Geometry: final body of the model. Coordinates: model frame, mm. Face numbers are marked on the shaded views. A direction names the side the tool comes from. Give positions to 0.01 mm unless a question says otherwise; leave off trailing zeros. Loops run counter-clockwise (first coordinate to the right, second up) from the corner with the lowest first, then second, coordinate; pieces in that order, holes last.
1. Section A-A, the plane y = 6. Output: boundary loops of the cut face in (x, z), then the cut area to 3 significant figures.
2. Section B-B, the plane y = -6.5. State how many separate pieces and enclosed holes the cut face has, then the cut area to 3 significant figures.
3. First-contact query: P1, Ø2, axis at y = -6, z = 19.5, coming from the +X side; P2, Ø15, axis at x = 0.5, z = -24.5, coming from the +Y side; P3, Ø1, axis at y = -6, z = -4, coming from the +X side. Flat tips, straight axial feed; report the tip coordinate or a pass-through.
4. Access query for the marked faces 1 and 2. Directions: +Z, -Z, +X, -X, +Y, -Y. A direction counts if a zero-diameter tool reaches every point of the face in a straight line with its end or side. Return the directions, or none.
5. Material intervals for line 1 along Z through (x, y) = (-6, 7); line 2 along X through (y, z) = (-7.5, 1.5); line 3 along X through (y, z) = (4.5, -15), sorted ascending.
6. Draft query along Y for the marked faces 3, 4, 5 and 6. Return one class per face: +Y half, -Y half, draft (parallel to the pull), parting line (faces both ways), or undercut.
from build123d import *

# Parameters (mm, degrees)
EXTRUDE_1_DEPTH     = 10
SHELL_2_T           = -1
SKETCH_8_W          = 4
SKETCH_8_H          = 7
EXTRUDE_3_DEPTH     = 5
SKETCH_9_R          = 3
CUT_EXTRUDE_1_DEPTH = 10


with BuildPart() as part:
    # 草图3 → 凸台-拉伸1 (new body)
    with BuildSketch(Plane(origin=(0, 0, 0), x_dir=(1, 0, 0), z_dir=(0, 1, 0))):
        Polygon((-25, 35), (-25, -25), (25, -25), (25, 35), (15, 45), (-15, 45), align=None)
    extrude(amount=EXTRUDE_1_DEPTH)


with BuildPart() as body_2:
    # 草图5 → 放样1 section 0
    with BuildSketch(Plane(origin=(0, 0, 0), x_dir=(1, 0, 0), z_dir=(0, 1, 0))):
        with BuildLine():
            Line((25, 35), (15, 45))
            Line((15, 45), (5, 35))
            Line((5, 35), (5, -25))
            Line((5, -25), (25, -25))
            Line((25, -25), (25, 35))
        make_face()
    # 草图6 → 放样1 section 1
    with BuildSketch(Plane(origin=(0, -10, 0), x_dir=(1, 0, 0), z_dir=(0, 1, 0))):
        with BuildLine():
            Line((22, -25), (8, -25))
            Line((8, -25), (8, 33.757359313))
            Line((8, 33.757359313), (15, 40.757359313))
            Line((15, 40.757359313), (22, 33.757359313))
            Line((22, 33.757359313), (22, -25))
        make_face()
    loft()


with BuildPart() as body_3:
    # 镜向2: mirrored copy
    add(body_2.part.mirror(Plane(origin=(0, 0, 0), x_dir=(0, 0, 1), z_dir=(1, 0, 0))))


with BuildPart() as part_1:
    add(part.part)

    # 相交1: read off the stored shape, not the designer's step
    # 相交1: union body 3, body 2
    add(body_3.part)
    add(body_2.part)

    # 草图7 → section 1 of loft_2
    with BuildSketch(Plane(origin=(0, 20, 0), x_dir=(1, 0, 0), z_dir=(0, 1, 0)), mode=Mode.PRIVATE) as loft_2_s1:
        with BuildLine():
            Line((-20, -24.480567501), (20, -24.480567501))
            Line((20, -24.480567501), (20, 25))
            Line((20, 25), (10, 35))
            Line((10, 35), (-10, 35))
            Line((-10, 35), (-20, 25))
            Line((-20, 25), (-20, -24.480567501))
        make_face()
    # loft from a face of the part (loft_2)
    loft([part_1.faces().sort_by_distance((0, 10, -9.068627451))[0], loft_2_s1.sketch])

    # 抽壳2
    shell_2_openings = [part_1.faces().sort_by_distance(p)[0] for p in [
        (0, 20, -4.10112168),
    ]]
    offset(amount=SHELL_2_T, openings=shell_2_openings, kind=Kind.INTERSECTION)

    # 草图8 → 凸台-拉伸3 (add)
    with BuildSketch(Plane(origin=(0, -9, 0), x_dir=(1, 0, 0), z_dir=(0, 1, 0))):
        with Locations((-16.744030651, -20.5)):
            Rectangle(SKETCH_8_W, SKETCH_8_H)
    extrude_3 = extrude(amount=EXTRUDE_3_DEPTH)

    # 草图9 → 切除-拉伸1 (cut)
    with BuildSketch(Plane.XY.offset(25)):
        with Locations((-16.744030651, -2.467331557)):
            Circle(SKETCH_9_R)
    cut_extrude_1 = extrude(amount=-CUT_EXTRUDE_1_DEPTH, mode=Mode.SUBTRACT)

    # 镜向3: 凸台-拉伸3, 切除-拉伸1 across plane
    add(extrude_3.mirror(Plane(origin=(0, 0, 0), x_dir=(0, 0, 1), z_dir=(1, 0, 0))))
    add(cut_extrude_1.mirror(Plane(origin=(0, 0, 0), x_dir=(0, 0, 1), z_dir=(1, 0, 0))), mode=Mode.SUBTRACT)


solid = part_1.part
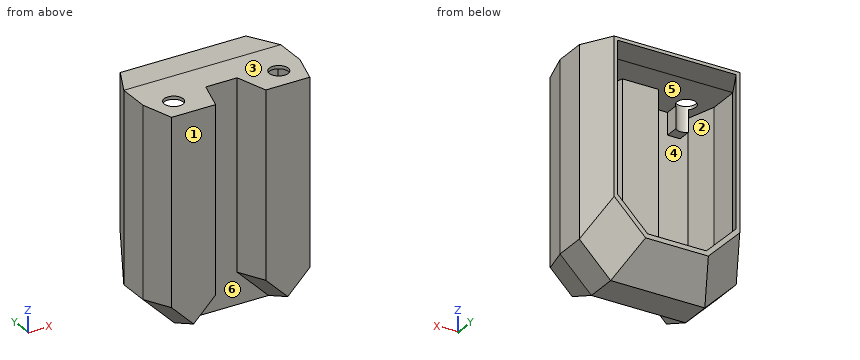
Answers below:
1. outline: (-25, -35) - (-15, -45) - (15, -45) - (25, -35) - (25, 25) - (-25, 25) - close; hole (-24, -34.59) - (-14.59, -44) - (14.59, -44) - (24, -34.59) - (24, 24) - (-24, 24) - close
1. area: 225 mm2
2. separate pieces: 2
2. enclosed holes: 2
2. area: 375 mm2
3. P1: stops at x = 23.5
3. P2: stops at y = 1
3. P3: stops at x = 23.35
4. face 1: +Z, -Z, +X, -X, -Y
4. face 2: none
5. line 1: z = -45 to -44, 24 to 25
5. line 2: x = -22.75 to -21.71, -8.29 to -7.25, 7.25 to 8.29, 21.71 to 22.75
5. line 3: x = -25 to -24, 24 to 25
6. face 3: draft
6. face 4: undercut
6. face 5: undercut
6. face 6: -Y half
